```python
from build123d import *

# Parameters (mm, degrees)
F0_W     = 76.2
F0_H     = 76.2
F1_DEPTH = 76.2
F2_W     = 75.00874
F2_H     = 74.538709
F3_DEPTH = 74.21626
F4_W     = 15.047822
F4_H     = 10.417721
F5_DEPTH = 23.8125
F7_DEPTH = 3.81


with BuildPart() as f1:
    # F0 (on Front) → F1 (new body)
    with BuildSketch(Plane.XZ):
        with Locations((-38.1, 38.1)):
            Rectangle(F0_W, F0_H)
    extrude(amount=F1_DEPTH)

    # F2 (on face) → F3 (cut)
    with BuildSketch(Plane.XZ.offset(76.2)):
        with Locations((-37.90061, 38.135625)):
            Rectangle(F2_W, F2_H)
    extrude(amount=-F3_DEPTH, mode=Mode.SUBTRACT)

    # F4 (on face) → F5 (cut)
    with BuildSketch(Plane.XZ.offset(1.98374)):
        with Locations((-36.997689, 16.123744)):
            Rectangle(F4_W, F4_H)
    extrude(amount=-F5_DEPTH, mode=Mode.SUBTRACT)

    # F6 (on face) → F7 (join)
    with BuildSketch(Plane.XZ.offset(1.98374)):
        with BuildLine():
            Line((-29.473778, 16.500985), (-29.473778, 14.723744))
            ThreePointArc((-29.473778, 14.723744), (-36.543118, 51.269556), (-45.348023, 15.102643))
            Line((-45.348023, 15.102643), (-45.348023, 16.92383))
            ThreePointArc((-45.348023, 16.92383), (-36.53353, 49.650186), (-29.473778, 16.500985))
        make_face()
    extrude(amount=F7_DEPTH)


solid = f1.part
```
Can you work these out from the model? Positions are in its coordinate system, mm. A direction names the side the tool comes from. Round coordinates to 2 decimals unless told otherwise and drop trailing zeros. Order: outer loops, then holes, each group sorted by start corner. A loop starts at its lowest first (then second) coordinate and runs counter-clockwise, first axis right, second up. Notation, with made-up numbers: (74.25, 65) -> (98.25, 65) arc R22 ccw to (98.25, 96) -> close; hole circle Ø9 at (8.5, -11). An arc over 180 degrees is marked (long way). Return JSON: item names as keys, results as strings. Group by question number.
1. Will this pin go through, and if not, where does the flat tip stop? pin 1 (4 mm diameter, centred on x = -35.5, z = 34, fed in from -Y).
2. If we section it at B-B, the plane z = 53: Write out the boundary of the cut face in (x, y), then the cut area to 3 significant figures.
3. We'd pull the mould along X, two halves only. Please class faces 4 (the face through (-39, -38, 0)), 5 (the face through (-35.82, -3.86, 51.24)), 6 (the face through (-76.2, -38, 38)): released by +X, released by -X, zero draft, split by the parting line, or undercut.
4. Which directions (+Z, -Z, +X, -X, +Y, -Y) give clear straight access to the entire face, cutting with the end or side of a thin tool? Please do faces 1 (the face through (0, -38, 38)), 2 (the face through (-75.405, -40, 38)), 3 (the face through (-44.522, -1, 16)).
5. I need wall thicknesses on line 1 (X direction, y = -68, z = 33.5); line 2 (Z direction, x = -46.5, y = -58.5); line 3 (Y direction, x = -45.5, z = 24). Which ranges of each line are inside material? Lowest first, please. Write a range as [from, to].
6. If we section it at D-D, the plane x = -38.5: Write out the boundary of the cut face in (y, z), then the cut area to 3 significant figures.
7. If we section it at A-A, the plane y = -16: Write out the boundary of the cut face in (x, z), then the cut area to 3 significant figures.
8. If we section it at C-C, the plane x = -11: Write out the boundary of the cut face in (y, z).
Output values:
{
 "1": {"pin 1": "y = -1.98"},
 "2": {"outline": "(-76.2, -76.2) -> (-75.4, -76.2) -> (-75.4, -1.98) -> (-0.4, -1.98) -> (-0.4, -76.2) -> (0, -76.2) -> (0, 0) -> (-76.2, 0) -> close", "area": "240 mm²"},
 "3": {"face 4": "zero draft", "face 5": "undercut", "face 6": "released by -X"},
 "4": {"face 1": "+Z, -Z, +X, +Y, -Y", "face 2": "-Y", "face 3": "+Y, -Y"},
 "5": {"line 1": "[-76.2, -75.4], [-0.4, 0]", "line 2": "[0, 0.87], [75.4, 76.2]", "line 3": "[-1.98, 0]"},
 "6": {"outline": "(-76.2, 0) -> (0, 0) -> (0, 10.91) -> (-1.98, 10.91) -> (-1.98, 0.87) -> (-76.2, 0.87) -> close; (-76.2, 75.4) -> (-1.98, 75.4) -> (-1.98, 51.22) -> (-5.79, 51.22) -> (-5.79, 49.59) -> (-1.98, 49.59) -> (-1.98, 21.33) -> (0, 21.33) -> (0, 76.2) -> (-76.2, 76.2) -> close", "area": "260 mm²"},
 "7": {"outline": "(-76.2, 0) -> (0, 0) -> (0, 76.2) -> (-76.2, 76.2) -> close; hole (-75.4, 0.87) -> (-0.4, 0.87) -> (-0.4, 75.4) -> (-75.4, 75.4) -> close", "area": "215 mm²"},
 "8": {"outline": "(-76.2, 0) -> (0, 0) -> (0, 76.2) -> (-76.2, 76.2) -> (-76.2, 75.4) -> (-1.98, 75.4) -> (-1.98, 0.87) -> (-76.2, 0.87) -> close"}
}
